Here's how the part is built. I have some questions about the finished solid (model axes, mm). A direction names the side the tool comes from. Give positions to 0.01 mm unless a question says otherwise; leave off trailing zeros. Loops run counter-clockwise (first coordinate to the right, second up) from the corner with the lowest first, then second, coordinate; pieces in that order, holes last.
Q1. If we section it at B-B (x = -46.5): Please give me the cut outline in (y, z).
Q2. If we section it at A-A (y = 2.75): Please give me the cut outline in (x, z) (3 decimals).
Q3. If we section it at D-D (y = 16.75): Please give me the cut outline in (x, z), plus the area to 3 significant figures.
Q4. I need wall thicknesses on line 1 (X direction, y = 1, z = -24.5) (3 decimals); line 2 (Z direction, x = 49.5, y = 2.5); line 3 (Y direction, x = -43, z = 47). Which ranges of each line are inside material? Lowest first, please.
Q5. Will these pins go through, and if not, where does the flat tip stop? P1, Ø1, axis at x = 17, z = -6.5, coming from the +Y side; P2, Ø1.5, axis at x = -46.5, z = -8.5, coming from the -Y side.
Q6. For faces 4 (the face through (-60, 10, 1)), 5 (the face through (-1, 4, 49.95)), which set-ups out of +Z, -Z, +X, -X, +Y, -Y let a thin tool reach every point of the face, with its end or its side?
Q7. We'd pull the mould along Z, two halves only. Please class faces 1 (the face through (-49.925, 4, 1)), 2 (the face through (-1, 10, 60)), 3 (the face through (-1, 10, -60)): +Z half, -Z half, draft (parallel to the pull), parting line (faces both ways), or undercut.
Q8. If we section it at C-C (z = 48): Please give me the cut outline in (x, y) (3 decimals), plus the area to 3 significant figures.
from build123d import *

# Parameters (mm, degrees)
SKETCH_2_W          = 120
SKETCH_2_H          = 120
EXTRUDE_1_DEPTH     = 20
SKETCH_4_W          = 99.85
SKETCH_4_H          = 99.9
CUT_EXTRUDE_1_DEPTH = 8


with BuildPart() as part:
    # 草图2 → 凸台-拉伸1 (new body)
    with BuildSketch(Plane(origin=(0, 0, 0), x_dir=(1, 0, 0), z_dir=(0, 1, 0))):
        Rectangle(SKETCH_2_W, SKETCH_2_H)
    extrude(amount=EXTRUDE_1_DEPTH)

    # 草图3 → 切除-旋转4 (revolve, cut)
    with BuildSketch(Plane.XY):
        with BuildLine():
            Line((-31.5, 43), (0, 43))
            Line((0, 43), (31.5, 43))
            ThreePointArc((31.5, 43), (0, 74.5), (-31.5, 43))
        make_face()
    revolve(axis=Axis((-31.5, 43, 0), (1, 0, 0)), mode=Mode.SUBTRACT)

    # 草图4 → 切除-拉伸1 (cut)
    with BuildSketch(Plane(origin=(0, 0, 0), x_dir=(1, 0, 0), z_dir=(0, 1, 0))):
        Rectangle(SKETCH_4_W, SKETCH_4_H)
    extrude(amount=CUT_EXTRUDE_1_DEPTH, mode=Mode.SUBTRACT)


solid = part.part
Check sheet entries:
1. outline: (0, -60) - (20, -60) - (20, 60) - (0, 60) - (0, 49.95) - (8, 49.95) - (8, -49.95) - (0, -49.95) - close
2. outline: (-60, -60) - (60, -60) - (60, 60) - (-60, 60) - close; hole (-49.925, -49.95) - (49.925, -49.95) - (49.925, 49.95) - (-49.925, 49.95) - close
3. outline: (-60, -60) - (60, -60) - (60, 60) - (-60, 60) - close; hole circle Ø34.82 at (0, 0)
3. area: 13,400 mm2
4. line 1: x = -60 to -49.925, 49.925 to 60
4. line 2: z = -60 to -49.95, 49.95 to 60
4. line 3: y = 8 to 20
5. P1: stops at y = 17.65
5. P2: stops at y = 8
6. face 4: +Z, -Z, -X, +Y, -Y
6. face 5: -Y
7. face 1: undercut
7. face 2: +Z half
7. face 3: -Z half
8. outline: (-60, 0) - (-49.925, 0) - (-49.925, 8) - (49.925, 8) - (49.925, 0) - (60, 0) - (60, 20) - (-60, 20) - close
8. area: 1,600 mm2
